from build123d import *

# Parameters (mm, degrees)
SKETCH_2_W             = 28
SKETCH_2_H             = 4.5
CUT_EXTRUDE_1_DEPTH    = 10
EXTRUDE_1_DEPTH        = 15
HOLE_WIZARD_M3_1_D     = 2.5
HOLE_WIZARD_M3_1_DEPTH = 4
HOLE_WIZARD_M3_1_TIP   = 0.751075774
CUT_EXTRUDE_START      = -20
CUT_EXTRUDE_2_DEPTH    = 20
HOLE_WIZARD_M4_1_D     = 3.3
HOLE_WIZARD_M4_1_DEPTH = 10.1
HOLE_WIZARD_M4_1_TIP   = 0.991420021
HOLE_WIZARD_M3_2_D     = 2.5


with BuildPart() as part:
    # 草图1 → 旋转1 (revolve)
    with BuildSketch(Plane.XY, mode=Mode.PRIVATE) as revolve_1_sk:
        Polygon((0, 0), (4.1, 0), (4.1, 6.7), (13.4, 6.7), (13.4, 8.7), (21, 8.7), (21, 10.2), (20, 10.2), (20, 11.2), (21, 11.2), (21, 12.2), (10, 12.2), (10, 13.2), (21, 13.2), (21, 20.4), (5, 20.4), (5, 21), (21, 21), (21, 34.7), (18.3, 38.7), (3.5, 38.7), (3.5, 43.7), (0, 43.7), align=None)
    revolve(revolve_1_sk.sketch.rotate(Axis((0, 43.7, 0), (0, -1, 0)), 90), axis=Axis((0, 43.7, 0), (0, -1, 0)))

    # 草图2 → 切除-拉伸1 (cut)
    with BuildSketch(Plane.XY.offset(21)):
        with Locations((0, 16.05)):
            Rectangle(SKETCH_2_W, SKETCH_2_H)
    extrude(amount=-CUT_EXTRUDE_1_DEPTH, mode=Mode.SUBTRACT)

    # 草图3 → 凸台-拉伸1 (add)
    with BuildSketch(Plane.XY.offset(11)):
        with BuildLine():
            Line((9.185056323, 18.053194417), (9.385056323, 18.053194417))
            ThreePointArc((9.385056323, 18.053194417), (11.385056323, 16.053194417), (9.385056323, 14.053194417))
            Line((9.385056323, 14.053194417), (9.185056323, 14.053194417))
            ThreePointArc((9.185056323, 14.053194417), (7.185056323, 16.053194417), (9.185056323, 18.053194417))
        make_face()
    extrude(amount=EXTRUDE_1_DEPTH)

    # M3 螺纹孔1
    with Locations(Plane(origin=(0, 38.7, 0), x_dir=(1, 0, 0), z_dir=(0, 1, 0))):
        with Locations((-6.5, 0), (6.5, 0)):
            Hole(HOLE_WIZARD_M3_1_D / 2, depth=HOLE_WIZARD_M3_1_DEPTH)
            with Locations((0, 0, -(HOLE_WIZARD_M3_1_DEPTH + HOLE_WIZARD_M3_1_TIP / 2))):  # 118° drill point
                Cone(0, HOLE_WIZARD_M3_1_D / 2, HOLE_WIZARD_M3_1_TIP, mode=Mode.SUBTRACT)

    # 草图7 → 旋转2 (revolve)
    with BuildSketch(Plane.XY, mode=Mode.PRIVATE) as revolve_2_sk:
        Polygon((0, -54.6), (5, -54.6), (5, -30.5), (8.275, -30.5), (8.275, -29.6), (13, -29.6), (13, -27.6), (21, -27.6), (21, 8.7), (0, 8.7), align=None)
    revolve(revolve_2_sk.sketch.rotate(Axis((0, 8.7, 0), (0, -1, 0)), 180), axis=Axis((0, 8.7, 0), (0, -1, 0)))

    # 草图8 → 切除-拉伸2 (cut)
    with BuildSketch(Plane.XZ.offset(54.6).offset(CUT_EXTRUDE_START)):
        with BuildLine():
            Line((-3, 4), (3, 4))
            ThreePointArc((3, 4), (0, 5), (-3, 4))
        make_face()
    extrude(amount=CUT_EXTRUDE_2_DEPTH, mode=Mode.SUBTRACT)

    # M4 螺纹孔1
    with Locations(Plane(origin=(0, -27.6, 0), x_dir=(-1, 0, 0), z_dir=(0, -1, 0))):
        with Locations((0, -17.5), (-17.5, 0), (0, 17.5), (17.5, 0)):
            Hole(HOLE_WIZARD_M4_1_D / 2, depth=HOLE_WIZARD_M4_1_DEPTH)
            with Locations((0, 0, -(HOLE_WIZARD_M4_1_DEPTH + HOLE_WIZARD_M4_1_TIP / 2))):  # 118° drill point
                Cone(0, HOLE_WIZARD_M4_1_D / 2, HOLE_WIZARD_M4_1_TIP, mode=Mode.SUBTRACT)

    # M3 螺纹孔2 (through all)
    with Locations(Plane(origin=(0, -44.6, 4), x_dir=(1, 0, 0), z_dir=(0, 0, 1))):
        with Locations((0, 0)):
            Hole(HOLE_WIZARD_M3_2_D / 2)


solid = part.part
Source: CAD feature listing. Evaluate the final solid. Frame: model axes, mm. A direction names the side the tool comes from. Coordinates: 2 decimals unless noted, no trailing zeros. Write each loop counter-clockwise with the first axis right and the second up, starting at its lowest first coordinate (ties: lowest second). Pieces come first, ordered by that corner, then holes. Notation, with made-up numbers: M 40,39 L 74,39 A4 ccw 74,43 Z; hole C 37.5,-30.75 d1. An arc over 180 degrees is marked long. Use a Markdown table: item, result.
1) Section B-B, the plane y = -44.6. Output: boundary loops of the cut face in (x, z), then the cut area to 3 significant figures.
Conclusion:
| item | result |
|---|---|
| outline | M -3,4 A5 ccw -1.25,-4.84 L -1.25,4 Z; M 1.25,-4.84 A5 ccw 3,4 L 1.25,4 Z |
| area | 52.1 mm^2 |
2) Mould query, pull axis Y, two halves, no side actions, for faces 6 (the conical face through (0.04, -16.68, 17.22)), 7 (the flat face through (0, 18.3, 15)), 8 (the conical face through (6.28, 34.08, -0.01)), 9 (the flat face through (4, 20.4, 4)). Classes: pulls with the +Y half, pulls with the -Y half, needs draft (parallel to the pull), parting line crosses it, or undercut.
Conclusion:
| item | result |
|---|---|
| face 6 | pulls with the -Y half |
| face 7 | undercut |
| face 8 | pulls with the +Y half |
| face 9 | undercut |
3) Reachability of faces 1 (the flat face through (9, 16, 26)), 2 (the cylindrical face through (7.186, 16.009, 18.395)), 3 (the cylindrical face through (-0.22, 20.704, -4.995)), 4 (the flat face through (-0.2, -29.6, 8.5)), 5 (the cylindrical face through (-5.25, 36.67, -0.05)) from +Z, -Z, +X, -X, +Y, -Y: full face, straight path, thin tool, end or side. Return the list, or none.
Conclusion:
| item | result |
|---|---|
| face 1 | +Z, +X, -X, +Y, -Y |
| face 2 | +Z |
| face 3 | none |
| face 4 | -Y |
| face 5 | +Y |
4) Section A-A, the plane y = -25.5. Output: boundary loops of the cut face in (x, z), then the cut area to 3 significant figures.
Conclusion:
| item | result |
|---|---|
| outline | C 0,0 d42; hole C -17.5,0 d3.3; hole C 0,-17.5 d3.3; hole C 0,17.5 d3.3; hole C 17.5,0 d3.3 |
| area | 1,350 mm^2 |
5) Section D-D, the plane z = -11.5. Give the number of separate pieces and of enclosed holes in the cut face, then the cut area to 3 significant figures.
Conclusion:
| item | result |
|---|---|
| separate pieces | 3 |
| enclosed holes | 0 |
| area | 2,280 mm^2 |
6) First-contact query: pin 1 Ø1.3 at (y, z) = (17, 14.5) entering from +X; pin 2 Ø5 at (x, y) = (2, 15.5) entering from +Z; pin 3 Ø5 at (y, z) = (17, 12.5) entering from -X; pin 4 Ø4 at (x, y) = (12.5, -33) entering from +Z. Flat tips, straight axial feed; report the tip coordinate or a pass-through.
Conclusion:
| item | result |
|---|---|
| pin 1 | stops at x = 15.79 |
| pin 2 | stops at z = 21 |
| pin 3 | stops at x = -18.47 |
| pin 4 | passes through |
7) Ray query, L1, parallel to Y at x = 2, z = 15; L2, parallel to Y at x = -15, z = 3.5; L3, parallel to Z at x = 0, y = -21. Return the intervals inside material, ascending.
Conclusion:
| item | result |
|---|---|
| L1 | y = -27.6 to 12.2, 13.2 to 13.8, 18.3 to 20.4, 21 to 38.7 |
| L2 | y = -27.6 to 12.2, 13.2 to 20.4, 21 to 38.7 |
| L3 | z = -21 to -19.15, -15.85 to 15.85, 19.15 to 21 |
8) Section C-C, the plane y = -5.5. Output: boundary loops of the cut face in (x, z), then the cut area to 3 significant figures.
Conclusion:
| item | result |
|---|---|
| outline | C 0,0 d42 |
| area | 1,390 mm^2 |
